```python
from build123d import *

# Parameters (mm, degrees)
BOSS_EXTRU_1_DEPTH      = 2
ESQUISSE4_R             = 0.75
ENL_V_MAT_EXTRU_2_DEPTH = 176.894862906
ENL_V_MAT_EXTRU_3_DEPTH = 4
CONG_2_R                = 1.35
ESQUISSE12_W            = 2
ESQUISSE12_H            = 5
BOSS_EXTRU_2_DEPTH      = 3
CONG_3_R                = 2
CONG_4_R                = 0.8
ESQUISSE13_W            = 5
ESQUISSE13_H            = 1.5
BOSS_EXTRU_3_DEPTH      = 6
CONG_5_R                = 1.5


with BuildPart() as part:
    # Esquisse2 → Boss.-Extru.1 (new body)
    with BuildSketch(Plane(origin=(0, 0, 0), x_dir=(0, 0, -1), z_dir=(1, 0, 0))):
        with BuildLine():
            Line((0, 0), (170.873171093, 0))
            ThreePointArc((170.873171093, 0), (174.177922559, 2.347343181), (173.049882129, 6.240789861))
            ThreePointArc((173.049882129, 6.240789861), (150.444362328, 18.689979585), (125, 23))
            ThreePointArc((125, 23), (61.450806457, 17.202138822), (0, 0))
        make_face()
    extrude(amount=BOSS_EXTRU_1_DEPTH)

    # Esquisse4 → Enlèv. mat.-Extru.2 (cut, through all)
    with BuildSketch(Plane(origin=(2, 0, 0), x_dir=(0, 0, -1), z_dir=(1, 0, 0))):
        with Locations((125, 21.5)):
            Circle(ESQUISSE4_R)
        with Locations((172.618958832, 3.328337296)):
            Circle(ESQUISSE4_R)
        with Locations((8, 1.25)):
            Circle(ESQUISSE4_R)
    extrude(amount=-ENL_V_MAT_EXTRU_2_DEPTH, mode=Mode.SUBTRACT)

    # Esquisse9 → Enlèv. mat.-Extru.3 (cut)
    with BuildSketch(Plane(origin=(0, 0, 0), x_dir=(0, 0, -1), z_dir=(1, 0, 0))):
        with BuildLine():
            Line((126.249998003, 1.5), (171.940959768, 1.5))
            ThreePointArc((171.940959768, 1.5), (170.669151645, 3.355758734), (171.992643995, 5.175018028))
            ThreePointArc((171.992643995, 5.175018028), (150.464605834, 17.100795028), (126.249998003, 21.497765776))
            Line((126.249998003, 21.497765776), (126.249998003, 1.5))
        make_face()
        with BuildLine():
            Line((9.933907961, 1.5), (60, 1.5))
            Line((60, 1.5), (60, 15.405547145))
            ThreePointArc((60, 15.405547145), (34.654135968, 9.627019927), (9.807619224, 1.981445651))
            ThreePointArc((9.807619224, 1.981445651), (9.886187662, 1.744768736), (9.933907961, 1.5))
        make_face()
        with BuildLine():
            Line((61.5, 1.5), (123.750001997, 1.5))
            Line((123.750001997, 1.5), (123.750001997, 21.497765776))
            ThreePointArc((123.750001997, 21.497765776), (92.494848054, 19.985907384), (61.5, 15.685935533))
            Line((61.5, 15.685935533), (61.5, 1.5))
        make_face()
    extrude(amount=ENL_V_MAT_EXTRU_3_DEPTH, mode=Mode.SUBTRACT)

    # Congé2
    cong_2_edges = [part.edges().sort_by_distance(p)[0] for p in [
        (1, 0, 0),
    ]]
    fillet(cong_2_edges, radius=CONG_2_R)

    # Esquisse12 → Boss.-Extru.2 (add)
    with BuildSketch(Plane.XZ):
        with Locations((1, -153.373171093)):
            Rectangle(ESQUISSE12_W, ESQUISSE12_H)
        with Locations((1, -24.612741703)):
            Rectangle(ESQUISSE12_W, ESQUISSE12_H)
    extrude(amount=BOSS_EXTRU_2_DEPTH)

    # Congé3
    cong_3_edges = [part.edges().sort_by_distance(p)[0] for p in [
        (1, 15.405547145, -60),
        (1, 21.497765776, -126.249998003),
        (1, 21.497765776, -123.750001997),
        (1, 15.685935533, -61.5),
    ]]
    fillet(cong_3_edges, radius=CONG_3_R)

    # Congé4
    cong_4_edges = [part.edges().sort_by_distance(p)[0] for p in [
        (1, 5.175018028, -171.992643995),
        (1, 1.5, -171.940959768),
    ]]
    fillet(cong_4_edges, radius=CONG_4_R)

    # Esquisse13 → Boss.-Extru.3 (add)
    with BuildSketch(Plane.ZY):
        with Locations((-153.373171093, 0.75)):
            Rectangle(ESQUISSE13_W, ESQUISSE13_H)
        with Locations((-24.612741703, 0.75)):
            Rectangle(ESQUISSE13_W, ESQUISSE13_H)
    extrude(amount=BOSS_EXTRU_3_DEPTH)

    # Congé5
    # the kernel refuses this fillet: 1.5 mm, written as the material it adds along each edge
    with BuildSketch(Plane(origin=(0, 1.5, -155.873171093), x_dir=(0, 0, -1), z_dir=(0, -1, 0)), Plane(origin=(0, 0, -150.873171093), x_dir=(0, 0, 1), z_dir=(0, 1, 0)), Plane(origin=(0, 1.5, -27.112741703), x_dir=(0, 0, -1), z_dir=(0, -1, 0)), Plane(origin=(0, 0, -22.112741703), x_dir=(0, 0, 1), z_dir=(0, 1, 0))) as cong_5_piece_1:
        with BuildLine():
            CenterArc((CONG_5_R, -CONG_5_R), CONG_5_R, 90, 90)
            Line((0, -CONG_5_R), (0, 0))
            Line((0, 0), (CONG_5_R, 0))
        make_face()
    extrude(amount=1.5)


solid = part.part
```
Check sheet for the modelled part. Datum: model origin and axes. Units: mm. A direction names the side the tool comes from. Round coordinates to 2 decimals unless told otherwise and drop trailing zeros. Write each loop counter-clockwise with the first axis right and the second up, starting at its lowest first coordinate (ties: lowest second). Pieces come first, ordered by that corner, then holes. Notation, with made-up numbers: (-25, -23) -> (-8, -23) arc R24 ccw to (-8, 4) -> close; hole circle Ø11 at (-5, 39). An arc over 180 degrees is marked (long way). One line per question, with ' | ' between items. Start each with the question number.
1. Scan lines: line 1 along Y through (x, z) = (1.4, -125); line 2 along Y through (x, z) = (-2, -151); line 3 along Y through (x, z) = (1.25, -100.5). Record each from-to range of solid material in increasing order. Write a range as from..to.
2. Set-up check for faces 1 (the face through (0, -1, -25)), 2 (the face through (2, 1, -96)), 3 (the face through (0.986, 9.402, -33.816)): record each of +Z, -Z, +X, -X, +Y, -Y from which the full face is reachable in a straight line by a thin tool's end or side.
3. Sectioned sample at A-A, the plane x = -4.5. Record the cut outline in (y, z).
4. Sectioned sample at B-B, the plane z = -88. Record the cut outline in (x, y), then the cut area to 3 significant figures.
5. Sectioned sample at C-C, the plane y = 10.5. Record the cut outline in (x, z), then the cut area to 3 significant figures.
6. Release check for a two-part mould opening along Y. For faces 4 (the face through (0.986, 2.29, -174.157)), 5 (the face through (0, -1, -153)), 6 (the face through (0.986, 20.008, -92.733)) record: +Y half, -Y half, draft (parallel to the pull), parting line (faces both ways), or undercut.
7. Depth check by flat-ended pin: pin 1 (2 mm diameter, centred on x = 1.5, y = -2, fed in from +Z); pin 2 (2 mm diameter, centred on x = 1, y = -2, fed in from -Z); pin 3 (1 mm diameter, centred on x = -1, z = -118.5, fed in from -Y); pin 4 (1.6 mm diameter, centred on x = 0.5, y = 5, fed in from -Z). Enter the tip coordinate at first touch or a pass-through.
Taken from the geometry:
1) line 1: y = 0..20.75, 22.25..23 | line 2: y = 0..1.5 | line 3: y = 0..1.5, 20.64..22.14
2) face 1: +Z, -Z, -X, -Y | face 2: +Z, -Z, +X, +Y, -Y | face 3: +X, -X
3) outline: (0, -155.87) -> (1.5, -155.87) -> (1.5, -150.87) -> (0, -150.87) -> close; (0, -27.11) -> (1.5, -27.11) -> (1.5, -22.11) -> (0, -22.11) -> close
4) outline: (0, 0) -> (2, 0) -> (2, 1.5) -> (0, 1.5) -> close; (0, 19.54) -> (2, 19.54) -> (2, 21.05) -> (0, 21.05) -> close | area: 6.02 mm^2
5) outline: (0, -167.13) -> (2, -167.13) -> (2, -164.33) -> (0, -164.33) -> close; (0, -126.25) -> (2, -126.25) -> (2, -123.75) -> (0, -123.75) -> close; (0, -61.5) -> (2, -61.5) -> (2, -60) -> (0, -60) -> close; (0, -37.98) -> (2, -37.98) -> (2, -32.14) -> (0, -32.14) -> close | area: 25.3 mm^2
6) face 4: parting line | face 5: draft | face 6: undercut
7) pin 1: stops at z = -22.11 | pin 2: stops at z = -155.87 | pin 3: passes through | pin 4: stops at z = -174.3
